```python
from build123d import *

# Parameters (mm, degrees)
SKETCH1_W             = 203.2
SKETCH1_H             = 177.8
BASE_DEPTH            = 4.826
CENTER_CUT_DEPTH      = 271.048829429
LEADING_EDGE_FILLET_R = 20.32
SKETCH3_W             = 4.826
SKETCH3_H             = 19.05
SIDE_SLOTS_DEPTH      = 271.048829429
SKETCH4_W             = 19.05
SKETCH4_H             = 4.826
REAR_SLOTS_DEPTH      = 271.048829429


with BuildPart() as part:
    # Sketch1 → Base (new body)
    with BuildSketch(Plane(origin=(0, 0, 0), x_dir=(1, 0, 0), z_dir=(0, 1, 0))):
        with Locations((101.6, 88.9)):
            Rectangle(SKETCH1_W, SKETCH1_H)
    extrude(amount=BASE_DEPTH)

    # Sketch2 → Center Cut (cut, through all)
    with BuildSketch(Plane(origin=(0, 4.826, 0), x_dir=(1, 0, 0), z_dir=(0, 1, 0))):
        Polygon((60.325, 89.870132361), (101.6, 66.04), (142.875, 89.870132361), (155.575, 177.8), (47.625, 177.8), align=None)
    extrude(amount=-CENTER_CUT_DEPTH, mode=Mode.SUBTRACT)

    # Leading Edge Fillet
    leading_edge_fillet_edges = [part.edges().sort_by_distance(p)[0] for p in [
        (47.625, 2.413, -177.8),
        (155.575, 2.413, -177.8),
    ]]
    fillet(leading_edge_fillet_edges, radius=LEADING_EDGE_FILLET_R)

    # Sketch3 → Side Slots (cut, through all)
    with BuildSketch(Plane(origin=(0, 4.826, 0), x_dir=(1, 0, 0), z_dir=(0, 1, 0))):
        with Locations((2.413, 107.95)):
            Rectangle(SKETCH3_W, SKETCH3_H)
        with Locations((2.413, 69.85)):
            Rectangle(SKETCH3_W, SKETCH3_H)
        with Locations((200.787, 69.85)):
            Rectangle(SKETCH3_W, SKETCH3_H)
        with Locations((200.787, 107.95)):
            Rectangle(SKETCH3_W, SKETCH3_H)
    extrude(amount=-SIDE_SLOTS_DEPTH, mode=Mode.SUBTRACT)

    # Sketch4 → Rear Slots (cut, through all)
    with BuildSketch(Plane(origin=(0, 4.826, 0), x_dir=(1, 0, 0), z_dir=(0, 1, 0))):
        with Locations((82.55, 2.413)):
            Rectangle(SKETCH4_W, SKETCH4_H)
        with Locations((120.65, 2.413)):
            Rectangle(SKETCH4_W, SKETCH4_H)
    extrude(amount=-REAR_SLOTS_DEPTH, mode=Mode.SUBTRACT)


solid = part.part
```
The listing builds one solid part. Answer for the finished solid, in the listing's coordinates (mm). A direction names the side the tool comes from. Give positions to 0.01 mm unless a question says otherwise; leave off trailing zeros. Order: outer loops, then holes, each group sorted by start corner. A loop starts at its lowest first (then second) coordinate and runs counter-clockwise, first axis right, second up. Notation, with made-up numbers: (-36.5, 3) -> (11.5, 3) arc R17 cw to (11.5, 10) -> close; hole circle Ø2 at (23.25, 7). An arc over 180 degrees is marked (long way). Answer as CSV lines item,"result". Start each with the question number.
Q1. Determine the mould class of faces 1 (the flat face through (166, 2, 0)), 2 (the flat face through (2, 2, -98.425)), 3 (the flat face through (2, 2, -79.375)), 4 (the cylindrical face through (43.18, 2.38, -172.97)) for opening direction Z: pulls with the +Z half, pulls with the -Z half, needs draft (parallel to the pull), parting line crosses it, or undercut.
Q2. A cutting plane is placed at B-B (z = -73.5). Determine the outline of the cut face in (x, y), then the cut area to 3 significant figures.
Q3. A cutting plane is placed at D-D (x = 78). Determine the outline of the cut face in (y, z), then the cut area to 3 significant figures.
Q4. A cutting plane is placed at C-C (x = 46). Determine the outline of the cut face in (y, z).
Q5. Which of the six approach directions +Z, -Z, +X, -X, +Y, -Y give full straight-line access (tool end or side, diameter ignored) to faces 5 (the flat face through (4.826, 2, -108)), 6 (the flat face through (111.125, 2, -2)), 7 (the flat face through (198.374, 2, -70)), 8 (the flat face through (80.674, 2.447, -78.122))?
Q6. Find the intervals of material crossed by L1, parallel to X at y = 4.45, z = -104.5; L2, parallel to X at y = 4.55, z = -119.5; L3, parallel to X at y = 4.55, z = -64, in increasing order.
Q7. Given pin 1 (1.4 mm diameter, centred on y = 1.5, z = -66.5, fed in from +X); pin 2 (1.5 mm diameter, centred on x = 162.5, y = 1.5, fed in from -Z); pin 3 (1.4 mm diameter, centred on x = 120.5, y = 2.5, fed in from +Z), each flat-ended and moving along its own axis, determine where each tip first touches the part or whether it passes through.
Q8. A cutting plane is placed at A-A (z = -140.5). Determine the outline of the cut face in (x, y).
Results found:
1,face 1,"pulls with the +Z half"
1,face 2,"undercut"
1,face 3,"undercut"
1,face 4,"pulls with the -Z half"
2,outline,"(4.83, 0) -> (88.68, 0) -> (88.68, 4.83) -> (4.83, 4.83) -> close; (114.52, 0) -> (198.37, 0) -> (198.37, 4.83) -> (114.52, 4.83) -> close"
2,area,"809 mm2"
3,outline,"(0, -79.67) -> (4.83, -79.67) -> (4.83, -4.83) -> (0, -4.83) -> close"
3,area,"361 mm2"
4,outline,"(0, -170.04) -> (4.83, -170.04) -> (4.83, 0) -> (0, 0) -> close"
5,face 5,"-X, +Y, -Y"
5,face 6,"+Z, +Y, -Y"
5,face 7,"+X, +Y, -Y"
5,face 8,"-Z, +Y, -Y"
6,L1,"4.83 to 58.21, 144.99 to 198.37"
6,L2,"0 to 56.05, 147.15 to 203.2"
6,L3,"4.83 to 198.37"
7,pin 1,"x = 198.37"
7,pin 2,"z = -175.21"
7,pin 3,"z = -4.83"
8,outline,"(0, 0) -> (53.01, 0) -> (53.01, 4.83) -> (0, 4.83) -> close; (150.19, 0) -> (203.2, 0) -> (203.2, 4.83) -> (150.19, 4.83) -> close"
